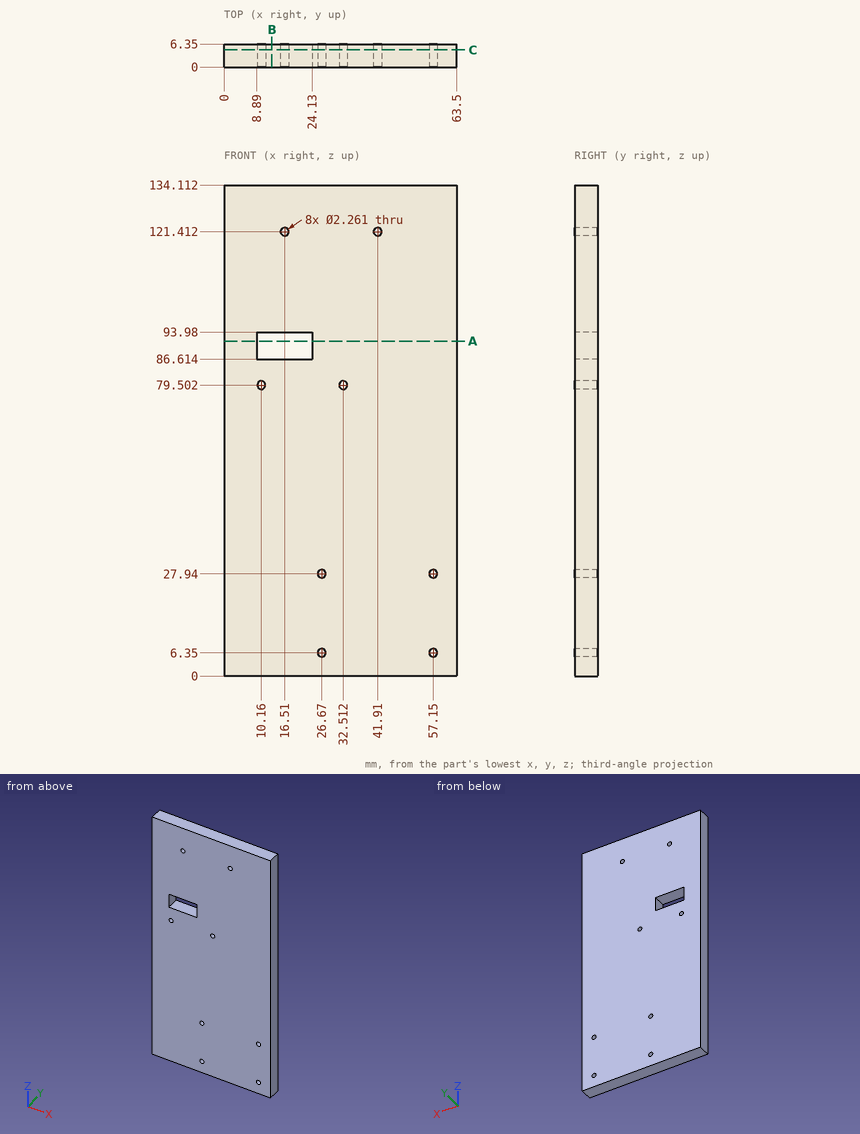
Job drawing, mm, ordinate dimensions from the low corner. One solid piece. Coordinates: 2 decimals unless noted, no trailing zeros. Order: outer loops, then holes, each group sorted by start corner. A loop starts at its lowest first (then second) coordinate and runs counter-clockwise, first axis right, second up. Notation, with made-up numbers: (36.5, 36.25) - (42.5, 36.25) arc R10 ccw to (42.5, 43.25) - close; hole circle Ø10 at (76.5, -18.5). An arc over 180 degrees is marked (long way). Return JSON: item names as keys, results as strings. Group by question number.
1) Saw through at A-A, the plane z = 91.5. Write the cut outline in (x, y).
2) Saw through at C-C, the plane y = 4.75. Count the separate pieces of the cut face and the enclosed holes in it, plus the area to 3 significant figures.
3) Probe line 1 (X direction, y = 4.25, z = 6.35); line 2 (Z direction, x = 10.16, y = 3.75); line 3 (Z direction, x = 57.15, y = 4). List the from-to ranges inside material, lowest first. Write a range as from..to.
4) Saw through at B-B, the plane x = 13. Write the cut outline in (y, z).
Values found:
{
 "1": {"outline": "(0, 0) - (8.89, 0) - (8.89, 6.35) - (0, 6.35) - close; (24.13, 0) - (63.5, 0) - (63.5, 6.35) - (24.13, 6.35) - close"},
 "2": {"separate pieces": "1", "enclosed holes": "9", "area": "8,370 mm²"},
 "3": {"line 1": "x = 0..25.54, 27.8..56.02, 58.28..63.5", "line 2": "z = 0..78.37, 80.63..86.61, 93.98..134.11", "line 3": "z = 0..5.22, 7.48..26.81, 29.07..134.11"},
 "4": {"outline": "(0, 0) - (6.35, 0) - (6.35, 86.61) - (0, 86.61) - close; (0, 93.98) - (6.35, 93.98) - (6.35, 134.11) - (0, 134.11) - close"}
}
